from build123d import *

# Parameters (mm, degrees)
BOSS_EXTRU_1_DEPTH      = 3
ESQUISSE2_R             = 15
ENL_V_MAT_EXTRU_1_DEPTH = 3
ESQUISSE3_W             = 100
ESQUISSE3_H             = 3
BOSS_EXTRU_2_DEPTH      = 20
ESQUISSE4_R             = 3.5
ENL_V_MAT_EXTRU_2_DEPTH = 3
ENL_V_MAT_EXTRU_3_DEPTH = 3
CONG_1_R                = 54
CONG_3_R                = 54
CONG_4_R                = 10
CONG_5_R                = 7


with BuildPart() as part:
    # Esquisse1 → Boss.-Extru.1 (new body)
    with BuildSketch(Plane.XY):
        Polygon((0, 0), (0, 60), (100, 60), (348.978261886, 50), (348.978261886, 10), (100, 0), align=None)
    extrude(amount=BOSS_EXTRU_1_DEPTH)

    # Esquisse2 → Enlèv. mat.-Extru.1 (cut)
    with BuildSketch(Plane.XY.offset(3)):
        with Locations((100, 25)):
            Circle(ESQUISSE2_R)
    extrude(amount=-ENL_V_MAT_EXTRU_1_DEPTH, mode=Mode.SUBTRACT)

    # Esquisse3 → Boss.-Extru.2 (add)
    with BuildSketch(Plane(origin=(0, 60, 0), x_dir=(1, 0, 0), z_dir=(0, 1, 0))):
        with Locations((50, -1.5)):
            Rectangle(ESQUISSE3_W, ESQUISSE3_H)
    extrude(amount=BOSS_EXTRU_2_DEPTH)

    # Esquisse4 → Enlèv. mat.-Extru.2 (cut)
    with BuildSketch(Plane.XY.offset(3)):
        with Locations((47, 70)):
            Circle(ESQUISSE4_R)
        with Locations((32, 70)):
            Circle(ESQUISSE4_R)
        with Locations((17, 70)):
            Circle(ESQUISSE4_R)
    extrude(amount=-ENL_V_MAT_EXTRU_2_DEPTH, mode=Mode.SUBTRACT)

    # Esquisse5 → Enlèv. mat.-Extru.3 (cut)
    with BuildSketch(Plane.XY.offset(3)):
        Polygon((100, 60), (57.10986159, 80), (100, 80), align=None)
    extrude(amount=-ENL_V_MAT_EXTRU_3_DEPTH, mode=Mode.SUBTRACT)

    # Congé1
    cong_1_edges = [part.edges().sort_by_distance(p)[0] for p in [
        (100, 60, 1.5),
        (57.10986159, 80, 1.5),
    ]]
    fillet(cong_1_edges, radius=CONG_1_R)

    # Congé3
    cong_3_edges = [part.edges().sort_by_distance(p)[0] for p in [
        (0, 0, 1.5),
    ]]
    fillet(cong_3_edges, radius=CONG_3_R)

    # Congé4
    cong_4_edges = [part.edges().sort_by_distance(p)[0] for p in [
        (348.978261886, 50, 1.5),
        (348.978261886, 10, 1.5),
    ]]
    fillet(cong_4_edges, radius=CONG_4_R)

    # Congé5
    cong_5_edges = [part.edges().sort_by_distance(p)[0] for p in [
        (0, 80, 1.5),
    ]]
    fillet(cong_5_edges, radius=CONG_5_R)


solid = part.part
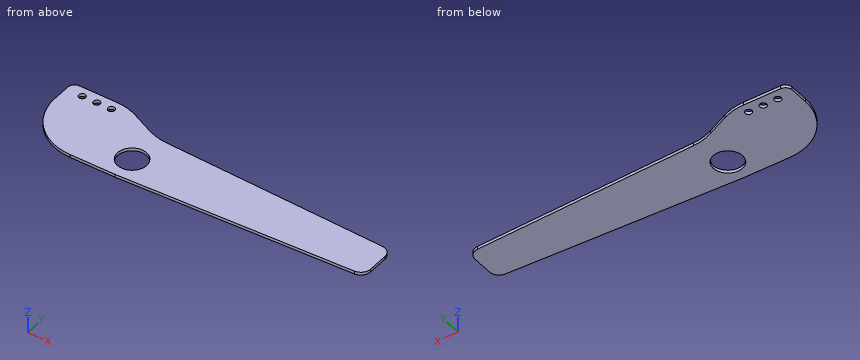
Can you work these out from the model? Positions are in its coordinate system, mm. Coordinates: 2 decimals unless noted, no trailing zeros. Write each loop counter-clockwise with the first axis right and the second up, starting at its lowest first coordinate (ties: lowest second). Pieces come first, ordered by that corner, then holes. Notation, with made-up numbers: (19.25, -9.75) - (62.25, -9.75) arc R19 cw to (62.25, 26.25) - close; hole circle Ø8 at (8, 78). An arc over 180 degrees is marked (long way). Return JSON: item names as keys, results as strings. Group by question number.
Item 1: I'm going to push flat-ended pins straight in: pin 1 Ø5.5 at (x, y) = (47, 70) entering from +Z; pin 2 Ø4 at (x, y) = (211, 52.5) entering from -Z. Where does each tip first touch, or does it pass through?
Item 2: If we section it at D-D (x = 32): Write out the boundary of the cut face in (y, z).
Item 3: If we section it at A-A (z = 1.6): Write out the boundary of the cut face in (x, y) (1 decimal), then the cut area to 3 significant figures.
Item 4: If we section it at B-B (y = 70): Write out the boundary of the cut face in (x, z).
Item 5: Please list where these lines run through material, in increasing order: probe 1 along X at (y, z) = (29, 2.7); probe 2 along Y at (x, z) = (32, 2.35); probe 3 along X at (y, z) = (19.5, 2.35).
Item 6: If we section it at C-C (y = 14): Write out the boundary of the cut face in (x, z), then the cut area to 3 significant figures.
Return value:
{
 "1": {"pin 1": "passes through", "pin 2": "stops at z = 0"},
 "2": {"outline": "(4.68, 0) - (66.5, 0) - (66.5, 3) - (4.68, 3) - close; (73.5, 0) - (80, 0) - (80, 3) - (73.5, 3) - close"},
 "3": {"outline": "(0, 54) arc R54 ccw to (54, 0) - (100, 0) - (339.4, 9.6) arc R10 ccw to (349, 19.6) - (349, 40.4) arc R10 ccw to (339.4, 50.4) - (110.8, 59.6) arc R54 cw to (90.2, 64.6) - (68, 74.9) arc R54 ccw to (45.1, 80) - (7, 80) arc R7 ccw to (0, 73) - close; hole circle Ø7 at (17, 70); hole circle Ø7 at (32, 70); hole circle Ø7 at (47, 70); hole circle Ø30 at (100, 25)", "area": "18,500 mm^2"},
 "4": {"outline": "(0, 0) - (13.5, 0) - (13.5, 3) - (0, 3) - close; (20.5, 0) - (28.5, 0) - (28.5, 3) - (20.5, 3) - close; (35.5, 0) - (43.5, 0) - (43.5, 3) - (35.5, 3) - close; (50.5, 0) - (78.55, 0) - (78.55, 3) - (50.5, 3) - close"},
 "5": {"probe 1": "x = 6.14 to 85.54, 114.46 to 348.98", "probe 2": "y = 4.68 to 66.5, 73.5 to 80", "probe 3": "x = 12.46 to 86.04, 113.96 to 348.98"},
 "6": {"outline": "(17.72, 0) - (89.8, 0) - (89.8, 3) - (17.72, 3) - close; (110.2, 0) - (347.26, 0) - (347.26, 3) - (110.2, 3) - close", "area": "927 mm^2"}
}
